Check sheet for the modelled part. Datum: model origin and axes. Units: mm. A direction names the side the tool comes from. Round coordinates to 2 decimals unless told otherwise and drop trailing zeros. Write each loop counter-clockwise with the first axis right and the second up, starting at its lowest first coordinate (ties: lowest second). Pieces come first, ordered by that corner, then holes. Notation, with made-up numbers: (56.5, 50) -> (88.5, 50) arc R12 ccw to (88.5, 57) -> close; hole circle Ø5 at (-29.75, 9). An arc over 180 degrees is marked (long way). One line per item, written item: value.
from build123d import *

# Parameters (mm, degrees)
F1_DEPTH  = 25.4
F2_R      = 6.35
F3_DEPTH  = 19.1426622189
F5_DEPTH  = 19.1426622189
F6_R      = 7.1994737013
F7_DEPTH  = 25.401
F9_DEPTH  = 25.4
F11_DEPTH = 19.1426622189


with BuildPart() as f1:
    # F0 (on Front) → F1 (new body)
    with BuildSketch(Plane.XZ):
        Polygon((-45.1743540521, 49.7133625326), (-70.570941653, 50.1297016121), (-70.570941653, 12.0297016121), (-0.7243540521, 12.0297016121), (-0.7243540521, 31.171363831), (-45.1743540521, 31.171363831), align=None)
    extrude(amount=F1_DEPTH)

    # F2 (on face) → F3 (cut, through all)
    with BuildSketch(Plane.XY.offset(31.171363831)):
        with Locations((-32.4743540521, -12.7)):
            Circle(F2_R)
        with Locations((-13.4243540521, -12.7)):
            Circle(F2_R)
    extrude(amount=-F3_DEPTH, mode=Mode.SUBTRACT)

    # F4 (on face) → F5 (cut, through all)
    with BuildSketch(Plane.XY.offset(31.171363831)):
        with BuildLine():
            Line((-13.4283372002, -6.3500012492), (-32.0889518764, -6.3617064471))
            ThreePointArc((-32.0889518764, -6.3617064471), (-27.8499728061, -8.3482649332), (-26.1243540521, -12.7))
            ThreePointArc((-26.1243540521, -12.7), (-27.9434136021, -17.1489412941), (-32.3583945682, -19.0489411242))
            Line((-32.3583945682, -19.0489411242), (-13.4247091757, -19.0499999901))
            ThreePointArc((-13.4247091757, -19.0499999901), (-19.774353793, -12.7018140123), (-13.4283372002, -6.3500012492))
        make_face()
    extrude(amount=-F5_DEPTH, mode=Mode.SUBTRACT)

    # F6 (on face) → F7 (cut, through all)
    with BuildSketch(Plane.XZ.offset(25.4)):
        with Locations((-58.0986022331, 36.3739425377)):
            Circle(F6_R)
    extrude(amount=-F7_DEPTH, mode=Mode.SUBTRACT)

    # F8 (on face) → F9 (cut)
    with BuildSketch(Plane.XZ.offset(25.4)):
        with BuildLine():
            ThreePointArc((-57.4608641224, 49.9147814938), (-50.0311914148, 47.4398241259), (-45.1743540521, 41.2968133537))
            Line((-45.1743540521, 41.2968133537), (-45.1743540521, 49.7133625326))
            Line((-45.1743540521, 49.7133625326), (-57.4608641224, 49.9147814938))
        make_face()
        with BuildLine():
            ThreePointArc((-70.570941653, 41.3884755726), (-65.5252942865, 47.5947800385), (-57.8726478526, 49.9215320724))
            Line((-57.8726478526, 49.9215320724), (-70.570941653, 50.1297016121))
            Line((-70.570941653, 50.1297016121), (-70.570941653, 41.3884755726))
        make_face()
    extrude(amount=-F9_DEPTH, mode=Mode.SUBTRACT)

    # F10 (on face) → F11 (cut, through all)
    with BuildSketch(Plane.XY.offset(31.171363831)):
        with BuildLine():
            ThreePointArc((-11.8059636609, 0), (-4.1674496382, -3.5171465582), (-0.7243540521, -11.1893241612))
            Line((-0.7243540521, -11.1893241612), (-0.7243540521, 0))
            Line((-0.7243540521, 0), (-11.8059636609, 0))
        make_face()
        with BuildLine():
            Line((-0.7243540521, -25.4), (-0.7243540521, -12.7))
            ThreePointArc((-0.7243540521, -12.7), (-4.4886377498, -21.6359661722), (-13.4247091757, -25.4))
            Line((-13.4247091757, -25.4), (-0.7243540521, -25.4))
        make_face()
    extrude(amount=-F11_DEPTH, mode=Mode.SUBTRACT)


solid = f1.part
Item 1: Material ranges on line 1 along Y through (x, z) = (-13, 27); line 2 along Z through (x, y) = (-13.5, -20.25); line 3 along X through (y, z) = (-2, 40), recorded low to high.
Result set:
line 1: -25.39 to -19.04, -6.36 to 0
line 2: 12.03 to 31.17
line 3: -70.57 to -64.32, -51.88 to -45.17
Item 2: Tool access check on faces 5 (the flat face through (-48, 0, 27)), 6 (the flat face through (-23, -4, 31.171)). Record the directions out of +Z, -Z, +X, -X, +Y, -Y that give a thin tool (end or side, any length) a straight path to the whole face; none if there is none.
Result set:
face 5: +Z, -Z, +X, -X, +Y
face 6: +Z, +X, +Y, -Y
Item 3: Sectioned sample at B-B (z = 20). Enter the section's corners in (x, y), then the cut area to 3 significant figures.
Result set:
outline: (-70.57, -25.4) -> (-13.42, -25.4) arc R12.85 ccw to (-0.72, -12.7) -> (-0.72, -11.19) arc R11.98 ccw to (-11.81, 0) -> (-70.57, 0) -> close; hole (-32.36, -19.05) -> (-13.42, -19.05) arc R6.35 ccw to (-13.43, -6.35) -> (-32.09, -6.36) arc R6.35 ccw (long way) to start
area: 1,340 mm^2
Item 4: Release check for a two-part mould opening along Y. For faces 1 (the cylindrical face through (-4.253, -3.432, 21.735)), 2 (the cylindrical face through (-7.076, -12.838, 21.735)), 3 (the cylindrical face through (-4.391, -21.537, 21.735)), 4 (the cylindrical face through (-38.82, -12.42, 21.73)) record: pulls with the +Y half, pulls with the -Y half, needs draft (parallel to the pull), parting line crosses it, or undercut.
Result set:
face 1: pulls with the +Y half
face 2: undercut
face 3: pulls with the -Y half
face 4: undercut
Item 5: Sectioned sample at C-C (x = -21.5). Enter the section's corners in (y, z), then the cut area to 3 significant figures.
Result set:
outline: (-25.4, 12.03) -> (-19.05, 12.03) -> (-19.05, 31.17) -> (-25.4, 31.17) -> close; (-6.36, 12.03) -> (0, 12.03) -> (0, 31.17) -> (-6.36, 31.17) -> close
area: 243 mm^2
Item 6: Sectioned sample at D-D (y = -1.5). Enter the section's corners in (x, z), then the cut area to 3 significant figures.
Result set:
outline: (-70.57, 12.03) -> (-6.82, 12.03) -> (-6.82, 31.17) -> (-45.17, 31.17) -> (-45.17, 41.3) arc R13.69 ccw to (-57.46, 49.91) -> (-57.87, 49.92) arc R13.69 ccw to (-70.57, 41.39) -> close; hole circle Ø14.4 at (-58.1, 36.37)
area: 1,470 mm^2
Item 7: Depth check by flat-ended pin: pin 1 (2 mm diameter, centred on x = -43, y = -6, fed in from +Z); pin 2 (8 mm diameter, centred on y = -21, z = 38, fed in from +X); pin 3 (3 mm diameter, centred on y = -3, z = 44.5, fed in from -X). Enter the tip coordinate at first touch or a pass-through.
Result set:
pin 1: z = 31.17
pin 2: x = -45.17
pin 3: x = -69.79
Item 8: Sectioned sample at A-A (y = -10.5). Enter the section's corners in (x, z), then the cut area to 3 significant figures.
Result set:
outline: (-70.57, 12.03) -> (-38.43, 12.03) -> (-38.43, 31.17) -> (-45.17, 31.17) -> (-45.17, 41.3) arc R13.69 ccw to (-57.46, 49.91) -> (-57.87, 49.92) arc R13.69 ccw to (-70.57, 41.39) -> close; (-7.47, 12.03) -> (-0.79, 12.03) -> (-0.79, 31.17) -> (-7.47, 31.17) -> close; hole circle Ø14.4 at (-58.1, 36.37)
area: 996 mm^2
